Source: three-view drawing plus pictorial views. Frame: mm from the lowest corner of the part. Give positions to 0.01 mm unless a question says otherwise; leave off trailing zeros. Loops run counter-clockwise (first coordinate to the right, second up) from the corner with the lowest first, then second, coordinate; pieces in that order, holes last.
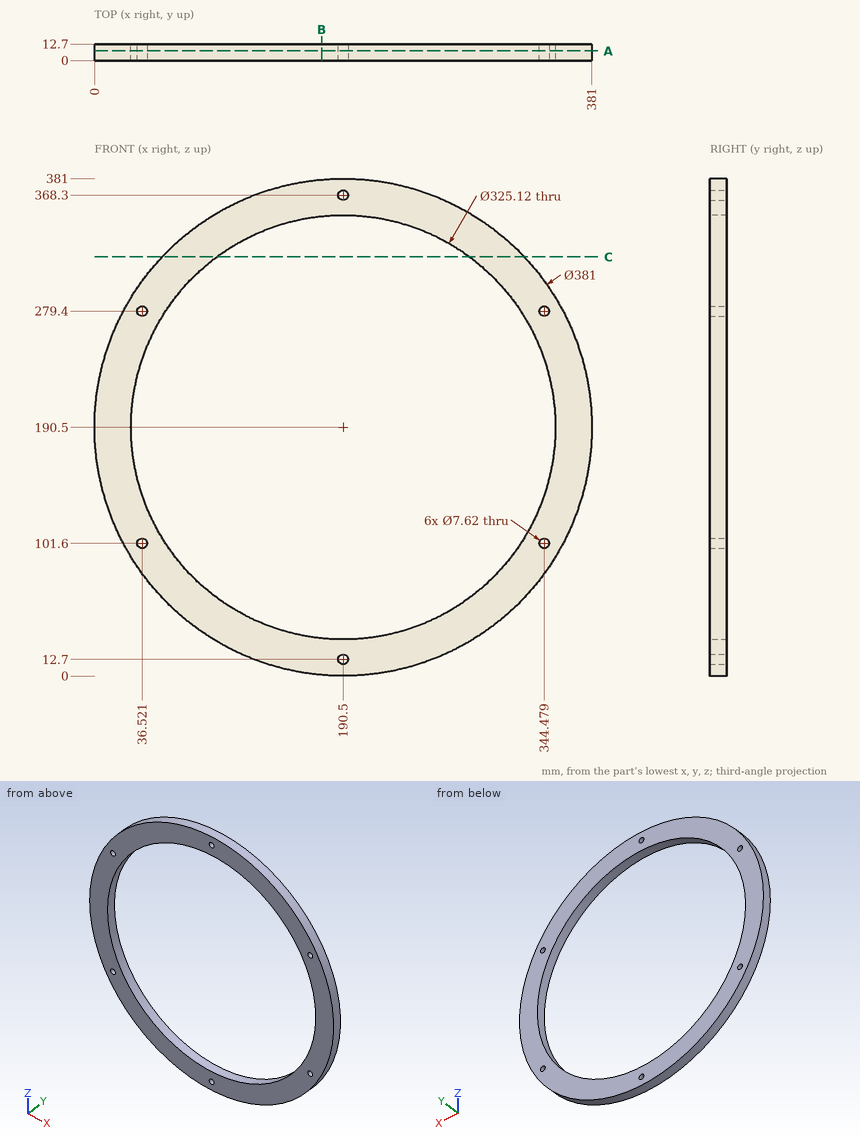
(1) Cut plane B-B (x = 174). Return the cut outline in (y, z), and give its area (3 significant figures).
Values follow:
outline: (0, 0.72) - (12.7, 0.72) - (12.7, 28.78) - (0, 28.78) - close; (0, 352.22) - (12.7, 352.22) - (12.7, 380.28) - (0, 380.28) - close
area: 713 mm2
(2) Ray query, probe 1 along Z at (x, y) = (190.5, 4.5); probe 2 along X at (y, z) = (6.75, 279.4) (1 decimal); probe 3 along X at (y, z) = (4.5, 332.5). Return the intervals inside material, ascending.
Values follow:
probe 1: z = 0 to 8.89, 16.51 to 27.94, 353.06 to 364.49, 372.11 to 381
probe 2: x = 22 to 32.7, 40.3 to 54.4, 326.6 to 340.7, 348.3 to 359
probe 3: x = 63.51 to 111.37, 269.63 to 317.49
(3) Pin query (flat end, axial travel): pin 1 Ø1 at (x, y) = (208, 11.5) entering from -Z; pin 2 Ø4 at (x, y) = (172.5, 1.5) entering from +Z; pin 3 Ø2 at (y, z) = (5.5, 189.5) entering from +X; pin 4 Ø1.5 at (x, y) = (314, 9.5) entering from -Z. Return the tip coordinate at first contact, or that it passes through.
Values follow:
pin 1: stops at z = 0.76
pin 2: stops at z = 380.33
pin 3: stops at x = 381
pin 4: stops at z = 44.82
(4) Cut plane C-C (z = 321). Return the cut outline in (x, y).
Values follow:
outline: (51.72, 0) - (93.57, 0) - (93.57, 12.7) - (51.72, 12.7) - close; (287.43, 0) - (329.28, 0) - (329.28, 12.7) - (287.43, 12.7) - close
(5) Cut plane A-A (y = 7.5). Return the cut outline in (x, z).
Values follow:
outline: circle Ø381 at (190.5, 190.5); hole circle Ø325.12 at (190.5, 190.5); hole circle Ø7.62 at (36.52, 101.6); hole circle Ø7.62 at (36.52, 279.4); hole circle Ø7.62 at (190.5, 12.7); hole circle Ø7.62 at (190.5, 368.3); hole circle Ø7.62 at (344.48, 101.6); hole circle Ø7.62 at (344.48, 279.4)
